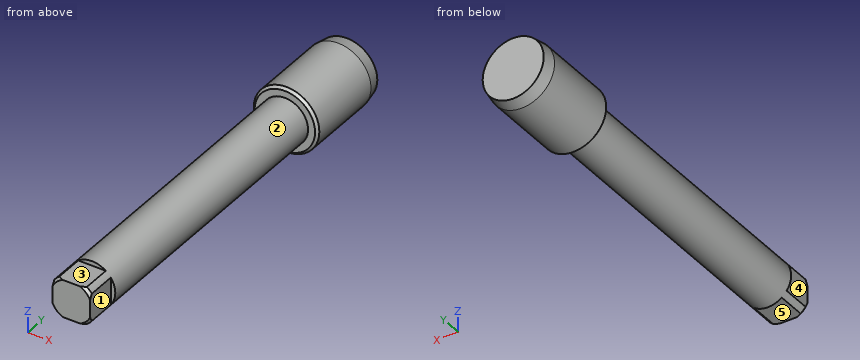
```python
from build123d import *

# Parameters (mm, degrees)
F0_R     = 9
F1_DEPTH = 160
F2_R     = 12.7
F3_DEPTH = 36
F4_SIZE2 = 0.881635
F4_SIZE  = 5
F5_SIZE  = 1
F6_W     = 18.961538
F6_H     = 20.995473
F6_W_2   = 14.5
F6_H_2   = 14.5
F7_DEPTH = 12


with BuildPart() as f1:
    # F0 (on Front) → F1 (new body)
    with BuildSketch(Plane.XZ):
        Circle(F0_R)
    extrude(amount=F1_DEPTH)

    # F2 (on Front) → F3 (join)
    with BuildSketch(Plane.XZ):
        Circle(F2_R)
    extrude(amount=F3_DEPTH)

    # F4
    f4_edges = [f1.edges().sort_by_distance(p)[0] for p in [
        (-12.7, 0, 0),
    ]]
    chamfer(f4_edges, length=F4_SIZE, length2=F4_SIZE2)

    # F5
    f5_edges = [f1.edges().sort_by_distance(p)[0] for p in [
        (-12.7, -36, 0),
        (-9, -160, 0),
    ]]
    chamfer(f5_edges, length=F5_SIZE)

    # F6 (on face) → F7 (cut)
    with BuildSketch(Plane.XZ.offset(160)):
        with Locations((0, -0.656108)):
            Rectangle(F6_W, F6_H)
        Rectangle(F6_W_2, F6_H_2, mode=Mode.SUBTRACT)
    extrude(amount=-F7_DEPTH, mode=Mode.SUBTRACT)


solid = f1.part
```
Check sheet for the modelled part. Datum: model origin and axes. Units: mm. Face numbers are marked on the shaded views. A direction names the side the tool comes from. Coordinates: 2 decimals unless noted, no trailing zeros. Loops run counter-clockwise (first coordinate to the right, second up) from the corner with the lowest first, then second, coordinate; pieces in that order, holes last. Notation, with made-up numbers: M 78.25,-5.5 L 83.25,-5.5 A32 cw 83.25,27.5 Z; hole C 80,-31.5 d8. An arc over 180 degrees is marked long. Answer as a JSON object with one key per item and string values.
1. Sectioned sample at C-C on y = -114. Record the cut outline in (x, z), and give its area (3 significant figures).
Outcome:
{"outline": "C 0,0 d18", "area": "254 mm²"}
2. Sectioned sample at A-A on z = 0. Record the cut outline in (x, y).
Outcome:
{"outline": "M -12.7,-35 L -11.7,-36 L -9,-36 L -9,-148 L -7.25,-148 L -7.25,-160 L 7.25,-160 L 7.25,-148 L 9,-148 L 9,-36 L 11.7,-36 L 12.7,-35 L 12.7,-5 L 11.82,0 L -11.82,0 L -12.7,-5 Z"}
3. Scan lines: L1, parallel to Z at x = 0, y = -41; L2, parallel to Y at x = 2.25, z = 10.75; L3, parallel to Z at x = 1, y = -153. Record each from-to range of solid material in increasing order. Write a range as from..to.
Outcome:
{"L1": "-9..9", "L2": "-36..0", "L3": "-7.25..7.25"}
4. Depth check by flat-ended pin: P1, Ø1.9, axis at x = 1, z = -8.5, coming from the -Y side; P2, Ø5.5, axis at x = 1.5, y = -156, coming from the +Z side; P3, Ø2, axis at x = -5.5, y = -88, coming from the -Z side; P4, Ø8, axis at x = 6, z = 9.5, coming from the -Y side. Enter the tip coordinate at first touch or a pass-through.
Outcome:
{"P1": "y = -148", "P2": "z = 7.25", "P3": "z = -7.79", "P4": "y = -160"}
5. Access from +Z, -Z, +X, -X, +Y, -Y to the whole of each face (thin tool, end or side, straight path). Record for the marked faces 1, 2, 3, 4 and 5.
Outcome:
{"face 1": "+Z, -Z, +X, -Y", "face 2": "-Y", "face 3": "+Z, +X, -X, -Y", "face 4": "+Z, -Z, -X, -Y", "face 5": "-Z, +X, -X, -Y"}
6. Sectioned sample at B-B on x = 0. Record the cut outline in (y, z).
Outcome:
{"outline": "M -160,-7.25 L -148,-7.25 L -148,-9 L -36,-9 L -36,-11.7 L -35,-12.7 L -5,-12.7 L 0,-11.82 L 0,11.82 L -5,12.7 L -35,12.7 L -36,11.7 L -36,9 L -148,9 L -148,7.25 L -160,7.25 Z"}
